from build123d import *

# Parameters (mm, degrees)
SKETCH1_R           = 2.5
SKETCH1_R_2         = 3.4
SKETCH1_R_3         = 2.75
BOSS_EXTRUDE1_DEPTH = 3.6
SKETCH3_W           = 22.86
SKETCH3_H           = 34.5
BOSS_EXTRUDE3_DEPTH = 1


with BuildPart() as part:
    # Sketch1 → Boss-Extrude1 (new body)
    with BuildSketch(Plane.XY):
        with BuildLine():
            Line((71.82, 0), (-71.82, 0))
            ThreePointArc((-71.82, 0), (-74.068599564, -0.931400436), (-75, -3.18))
            Line((-75, -3.18), (-75, -56.82))
            ThreePointArc((-75, -56.82), (-74.068599564, -59.068599564), (-71.82, -60))
            Line((-71.82, -60), (-18.28, -60))
            ThreePointArc((-18.28, -60), (-12.623145751, -62.343145751), (-10.28, -68))
            Line((-10.28, -68), (-10.28, -73.82))
            ThreePointArc((-10.28, -73.82), (-9.348599564, -76.068599564), (-7.1, -77))
            Line((-7.1, -77), (56.9, -77))
            ThreePointArc((56.9, -77), (59.148599564, -76.068599564), (60.08, -73.82))
            Line((60.08, -73.82), (60.08, -68))
            ThreePointArc((60.08, -68), (62.423145751, -62.343145751), (68.08, -60))
            Line((68.08, -60), (71.82, -60))
            ThreePointArc((71.82, -60), (74.068599564, -59.068599564), (75, -56.82))
            Line((75, -56.82), (75, -3.18))
            ThreePointArc((75, -3.18), (74.068599564, -0.931400436), (71.82, 0))
        make_face()
        with Locations((-35, -45)):
            Circle(SKETCH1_R, mode=Mode.SUBTRACT)
        with Locations((0, -10)):
            Circle(SKETCH1_R, mode=Mode.SUBTRACT)
        with Locations((-0.1, -65)):
            Circle(SKETCH1_R_2, mode=Mode.SUBTRACT)
        with Locations((49.9, -65)):
            Circle(SKETCH1_R_2, mode=Mode.SUBTRACT)
        with Locations((33.08, -72.5)):
            Circle(SKETCH1_R_3, mode=Mode.SUBTRACT)
        with Locations((18.22, -72.5)):
            Circle(SKETCH1_R_3, mode=Mode.SUBTRACT)
        with Locations((33.08, -47.5)):
            Circle(SKETCH1_R_3, mode=Mode.SUBTRACT)
    extrude(amount=BOSS_EXTRUDE1_DEPTH)

    # Sketch3 → Boss-Extrude3 (add)
    with BuildSketch(Plane(origin=(0, 0, 0), x_dir=(-1, 0, 0), z_dir=(0, 0, -1))):
        with Locations((-25.65, -59.75)):
            Rectangle(SKETCH3_W, SKETCH3_H)
    extrude(amount=-BOSS_EXTRUDE3_DEPTH)


solid = part.part
Verification items for the finished model (mm, model axes). A direction names the side the tool comes from. Give positions to 0.01 mm unless a question says otherwise; leave off trailing zeros. Write each loop counter-clockwise with the first axis right and the second up, starting at its lowest first coordinate (ties: lowest second). Pieces come first, ordered by that corner, then holes. Notation, with made-up numbers: M 41,2.25 L 46,2.25 A14 ccw 46,23.25 Z; hole C 15,42 d9. An arc over 180 degrees is marked long. Use CSV: the item, a comma, the result in double quotes.
1) Cross-section at C-C (z = 1.85). Enter the section's corners in (x, y).
Final values:
outline,"M -75,-56.82 A3.18 ccw -71.82,-60 L -18.28,-60 A8 cw -10.28,-68 L -10.28,-73.82 A3.18 ccw -7.1,-77 L 56.9,-77 A3.18 ccw 60.08,-73.82 L 60.08,-68 A8 cw 68.08,-60 L 71.82,-60 A3.18 ccw 75,-56.82 L 75,-3.18 A3.18 ccw 71.82,0 L -71.82,0 A3.18 ccw -75,-3.18 Z; hole C -35,-45 d5; hole C -0.1,-65 d6.8; hole C 0,-10 d5; hole C 18.22,-72.5 d5.5; hole C 33.08,-72.5 d5.5; hole C 33.08,-47.5 d5.5; hole C 49.9,-65 d6.8"
2) Release check for a two-part mould opening along X. For faces 5 (the face through (31.053, -70.641, 2.282)), 6 (the face through (-74.093, -59.044, 1.775)), 7 (the face through (70, -60, 2)) record: released by +X, released by -X, zero draft, split by the parting line, or undercut.
Final values:
face 5,"undercut"
face 6,"released by -X"
face 7,"zero draft"
3) Cross-section at D-D (x = 18.22). Enter the section's corners in (y, z).
Final values:
outline,"M -77,0 L 0,0 L 0,3.6 L -69.75,3.6 L -69.75,1 L -75.25,1 L -75.25,3.6 L -77,3.6 Z"
4) Go/stop test with flat-tipped pins: pin 1 Ø10 at (x, y) = (-24, -47) entering from -Z; pin 2 Ø3 at (x, y) = (-35, -45) entering from +Z; pin 3 Ø1.8 at (x, z) = (70, 1.5) entering from -Y; pin 4 Ø3 at (x, y) = (32, -73) entering from +Z. Record where each tip stops, or that it passes through.
Final values:
pin 1,"z = 0"
pin 2,"through"
pin 3,"y = -60"
pin 4,"z = 1"
5) Access from +Z, -Z, +X, -X, +Y, -Y to the whole of each face (thin tool, end or side, straight path). Record for faces 1 (the face through (60.08, -71, 2)), 2 (the face through (-10.28, -71, 2)), 3 (the face through (33, -72, 1)), 4 (the face through (1, 0, 2)).
Final values:
face 1,"+Z, -Z, +X, -Y"
face 2,"+Z, -Z, -X, -Y"
face 3,"+Z"
face 4,"+Z, -Z, +X, -X, +Y"
6) Material ranges on line 1 along X through (y, z) = (-72.5, 2); line 2 along Y through (x, z) = (33.08, 2.85); line 3 along Y through (x, z) = (-0.1, 1.8), recorded low to high.
Final values:
line 1,"-10.28 to 15.47, 20.97 to 30.33, 35.83 to 60.08"
line 2,"-77 to -75.25, -69.75 to -50.25, -44.75 to 0"
line 3,"-77 to -68.4, -61.6 to -12.5, -7.5 to 0"
7) Cross-section at A-A (x = -35). Enter the section's corners in (y, z).
Final values:
outline,"M -60,0 L -47.5,0 L -47.5,3.6 L -60,3.6 Z; M -42.5,0 L 0,0 L 0,3.6 L -42.5,3.6 Z"
8) Cross-section at B-B (y = -10). Enter the section's corners in (x, z), plus the area to 3 significant figures.
Final values:
outline,"M -75,0 L -2.5,0 L -2.5,3.6 L -75,3.6 Z; M 2.5,0 L 75,0 L 75,3.6 L 2.5,3.6 Z"
area,"522 mm²"
